Could you check a few things on this model? Use its own coordinates, in mm. Face numbers are marked on the shaded views. A direction names the side the tool comes from. Coordinates: 2 decimals unless noted, no trailing zeros. Write each loop counter-clockwise with the first axis right and the second up, starting at its lowest first coordinate (ties: lowest second). Pieces come first, ordered by that corner, then holes.
Item 1: I want a section at C-C on x = -18.5. Please give me the cut outline in (y, z).
Item 2: Which directions (+Z, -Z, +X, -X, +Y, -Y) give clear straight access to the entire face, cutting with the end or side of a thin tool? Please do the marked faces 4 and 5.
Item 3: If I drill on probe 1 along X at (y, z) = (-8, -2.25); probe 2 along X at (y, z) = (17, -2.5); probe 3 along Y at (x, z) = (-27.5, -4), over which ranges is the centre line in solid material (lowest first)?
Item 4: I want a section at D-D on y = -13. Please give me the cut outline in (x, z), then the cut area to 3 significant figures.
Item 5: Thinking about a two-plate mould opening in Y: for the marked faces 1, 2 and 3, which applies, +Y half, -Y half, draft (parallel to the pull), parting line (faces both ways), or undercut?
Item 6: For P1, Ø1.6, axis at y = 20, z = -4.5, coming from the +X side; P2, Ø10, axis at x = 45, y = -15.5, coming from the -Z side; P3, Ø1, axis at x = 29, y = 20, coming from the -Z side; P4, Ø1.5, axis at x = 4, z = -1, coming from the +Y side, each with a flat end and sliding along its axis, tell me the tip position at first contact or that it passes through.
Item 7: I want a section at B-B on y = -6. Please give me the cut outline in (x, z).
Item 8: I want a section at A-A on x = 8. Please give me the cut outline in (y, z).
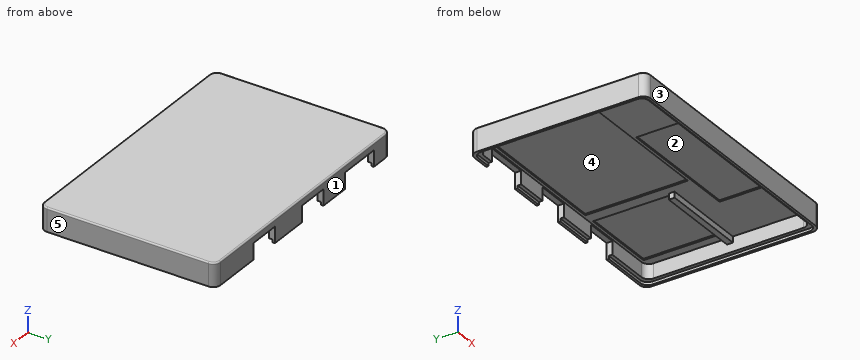
from build123d import *

# Parameters (mm, degrees)
SKETCH_1_W          = 90
SKETCH_1_H          = 60
EXTRUDE_1_DEPTH     = 2
SKETCH_2_W          = 50
SKETCH_2_H          = 35
EXTRUDE_2_DEPTH     = 1
SKETCH_3_W          = 14
SKETCH_3_H          = 13
EXTRUDE_3_DEPTH     = 10
SKETCH_4_W          = 10
SKETCH_4_H          = 12
EXTRUDE_4_DEPTH     = 5
SKETCH_5_W          = 26
SKETCH_5_H          = 26
EXTRUDE_5_DEPTH     = 1
SKETCH_6_W          = 10
SKETCH_6_H          = 10
EXTRUDE_6_DEPTH     = 7
SKETCH_7_W          = 43
SKETCH_7_H          = 18
EXTRUDE_7_DEPTH     = 1
SKETCH_8_W          = 2
SKETCH_8_H          = 60
EXTRUDE_8_DEPTH     = 5
SKETCH_9_W          = 88
SKETCH_9_H          = 2
EXTRUDE_9_DEPTH     = 5
SKETCH_10_W         = 2
SKETCH_10_H         = 58
EXTRUDE_10_DEPTH    = 5
SKETCH_11_W         = 86
SKETCH_11_H         = 2
EXTRUDE_11_DEPTH    = 5
SKETCH_12_W         = 0.8
SKETCH_12_H         = 60
EXTRUDE_12_DEPTH    = 1
SKETCH_13_W         = 89.2
SKETCH_13_H         = 0.8
EXTRUDE_13_DEPTH    = 1
SKETCH_14_W         = 0.8
SKETCH_14_H         = 59.2
EXTRUDE_14_DEPTH    = 1
SKETCH_15_W         = 88.4
SKETCH_15_H         = 0.8
EXTRUDE_15_DEPTH    = 1
SKETCH_16_W         = 11
SKETCH_16_H         = 8
CUT_EXTRUDE_2_DEPTH = 34
SKETCH_17_W         = 11
SKETCH_17_H         = 6
CUT_EXTRUDE_3_DEPTH = 34
SKETCH_18_W         = 15
SKETCH_18_H         = 11
CUT_EXTRUDE_4_DEPTH = 34
SKETCH_19_W         = 30
SKETCH_19_H         = 2
EXTRUDE_16_DEPTH    = 2
SKETCH_20_W         = 43
SKETCH_20_H         = 18
CUT_EXTRUDE_5_DEPTH = 1.5
SKETCH_21_W         = 26
SKETCH_21_H         = 26
CUT_EXTRUDE_6_DEPTH = 1.5
SKETCH_22_W         = 50
SKETCH_22_H         = 35
CUT_EXTRUDE_7_DEPTH = 1.5
FILLET_1_R          = 2.5
FILLET_2_R          = 2.5
FILLET_3_R          = 0.5


with BuildPart() as part:
    # Эскиз1 → Бобышка-Вытянуть1 (new body)
    with BuildSketch(Plane.XY):
        with Locations((11.347826087, -8.739130435)):
            Rectangle(SKETCH_1_W, SKETCH_1_H)
    extrude(amount=EXTRUDE_1_DEPTH)

    # Эскиз2 → Бобышка-Вытянуть2 (add)
    with BuildSketch(Plane(origin=(0, 0, 0), x_dir=(-1, 0, 0), z_dir=(0, 0, -1))):
        with Locations((3.652173913, 0.760869565)):
            Rectangle(SKETCH_2_W, SKETCH_2_H)
    extrude(amount=EXTRUDE_2_DEPTH)

    # Эскиз3 → Бобышка-Вытянуть3 (add)
    with BuildSketch(Plane(origin=(0, 0, -1), x_dir=(-1, 0, 0), z_dir=(0, 0, -1))):
        with Locations((17.652173913, 5.760869565)):
            Rectangle(SKETCH_3_W, SKETCH_3_H)
    extrude(amount=EXTRUDE_3_DEPTH)

    # Эскиз4 → Бобышка-Вытянуть4 (add)
    with BuildSketch(Plane(origin=(0, 0, -1), x_dir=(-1, 0, 0), z_dir=(0, 0, -1))):
        with Locations((-6.347826087, 15.260869565)):
            Rectangle(SKETCH_4_W, SKETCH_4_H)
    extrude(amount=EXTRUDE_4_DEPTH)

    # Эскиз5 → Бобышка-Вытянуть5 (add)
    with BuildSketch(Plane(origin=(0, 0, 0), x_dir=(-1, 0, 0), z_dir=(0, 0, -1))):
        with Locations((-38.347826087, 5.260869565)):
            Rectangle(SKETCH_5_W, SKETCH_5_H)
    extrude(amount=EXTRUDE_5_DEPTH)

    # Эскиз6 → Бобышка-Вытянуть6 (add)
    with BuildSketch(Plane(origin=(0, 0, -1), x_dir=(-1, 0, 0), z_dir=(0, 0, -1))):
        with Locations((-31.347826087, 14.260869565)):
            Rectangle(SKETCH_6_W, SKETCH_6_H)
    extrude(amount=EXTRUDE_6_DEPTH)

    # Эскиз7 → Бобышка-Вытянуть7 (add)
    with BuildSketch(Plane(origin=(0, 0, 0), x_dir=(-1, 0, 0), z_dir=(0, 0, -1))):
        with Locations((-14.606181905, -26.739130435)):
            Rectangle(SKETCH_7_W, SKETCH_7_H)
    extrude(amount=EXTRUDE_7_DEPTH)

    # Эскиз8 → Бобышка-Вытянуть8 (add)
    with BuildSketch(Plane(origin=(0, 0, 0), x_dir=(-1, 0, 0), z_dir=(0, 0, -1))):
        with Locations((-55.347826087, -8.739130435)):
            Rectangle(SKETCH_8_W, SKETCH_8_H)
    extrude(amount=EXTRUDE_8_DEPTH)

    # Эскиз9 → Бобышка-Вытянуть9 (add)
    with BuildSketch(Plane(origin=(0, 0, 0), x_dir=(-1, 0, 0), z_dir=(0, 0, -1))):
        with Locations((-10.347826087, -37.739130435)):
            Rectangle(SKETCH_9_W, SKETCH_9_H)
    extrude(amount=EXTRUDE_9_DEPTH)

    # Эскиз10 → Бобышка-Вытянуть10 (add)
    with BuildSketch(Plane(origin=(0, 0, 0), x_dir=(-1, 0, 0), z_dir=(0, 0, -1))):
        with Locations((32.652173913, -7.739130435)):
            Rectangle(SKETCH_10_W, SKETCH_10_H)
    extrude(amount=EXTRUDE_10_DEPTH)

    # Эскиз11 → Бобышка-Вытянуть11 (add)
    with BuildSketch(Plane(origin=(0, 0, 0), x_dir=(-1, 0, 0), z_dir=(0, 0, -1))):
        with Locations((-11.347826087, 20.260869565)):
            Rectangle(SKETCH_11_W, SKETCH_11_H)
    extrude(amount=EXTRUDE_11_DEPTH)

    # Эскиз12 → Бобышка-Вытянуть12 (add)
    with BuildSketch(Plane(origin=(0, 0, -5), x_dir=(-1, 0, 0), z_dir=(0, 0, -1))):
        with Locations((-55.947826087, -8.739130435)):
            Rectangle(SKETCH_12_W, SKETCH_12_H)
    extrude(amount=EXTRUDE_12_DEPTH)

    # Эскиз13 → Бобышка-Вытянуть13 (add)
    with BuildSketch(Plane(origin=(0, 0, -5), x_dir=(-1, 0, 0), z_dir=(0, 0, -1))):
        with Locations((-10.947826087, -38.339130435)):
            Rectangle(SKETCH_13_W, SKETCH_13_H)
    extrude(amount=EXTRUDE_13_DEPTH)

    # Эскиз14 → Бобышка-Вытянуть14 (add)
    with BuildSketch(Plane(origin=(0, 0, -5), x_dir=(-1, 0, 0), z_dir=(0, 0, -1))):
        with Locations((33.252173913, -8.339130435)):
            Rectangle(SKETCH_14_W, SKETCH_14_H)
    extrude(amount=EXTRUDE_14_DEPTH)

    # Эскиз15 → Бобышка-Вытянуть15 (add)
    with BuildSketch(Plane(origin=(0, 0, -5), x_dir=(-1, 0, 0), z_dir=(0, 0, -1))):
        with Locations((-11.347826087, 20.860869565)):
            Rectangle(SKETCH_15_W, SKETCH_15_H)
    extrude(amount=EXTRUDE_15_DEPTH)

    # Эскиз16 → Вырез-Вытянуть2 (cut)
    with BuildSketch(Plane.XZ.offset(-9.260869565)):
        with Locations((31.347826087, -4.5)):
            Rectangle(SKETCH_16_W, SKETCH_16_H)
    extrude(amount=-CUT_EXTRUDE_2_DEPTH, mode=Mode.SUBTRACT)

    # Эскиз17 → Вырез-Вытянуть3 (cut)
    with BuildSketch(Plane.XZ.offset(-9.260869565)):
        with Locations((6.347826087, -3.5)):
            Rectangle(SKETCH_17_W, SKETCH_17_H)
    extrude(amount=-CUT_EXTRUDE_3_DEPTH, mode=Mode.SUBTRACT)

    # Эскиз18 → Вырез-Вытянуть4 (cut)
    with BuildSketch(Plane.XZ.offset(0.739130435)):
        with Locations((-17.652173913, -6)):
            Rectangle(SKETCH_18_W, SKETCH_18_H)
    extrude(amount=-CUT_EXTRUDE_4_DEPTH, mode=Mode.SUBTRACT)

    # Эскиз19 → Бобышка-Вытянуть16 (add)
    with BuildSketch(Plane(origin=(0, 0, 0), x_dir=(-1, 0, 0), z_dir=(0, 0, -1))):
        with Locations((-39.347826087, -9.239130435)):
            Rectangle(SKETCH_19_W, SKETCH_19_H)
    extrude(amount=EXTRUDE_16_DEPTH)

    # Эскиз20 → Вырез-Вытянуть5 (cut)
    with BuildSketch(Plane(origin=(0, 0, -1), x_dir=(-1, 0, 0), z_dir=(0, 0, -1))):
        with Locations((-14.606181905, -26.739130435)):
            Rectangle(SKETCH_20_W, SKETCH_20_H)
    extrude(amount=-CUT_EXTRUDE_5_DEPTH, mode=Mode.SUBTRACT)

    # Эскиз21 → Вырез-Вытянуть6 (cut)
    with BuildSketch(Plane(origin=(0, 0, -1), x_dir=(-1, 0, 0), z_dir=(0, 0, -1))):
        with Locations((-38.347826087, 5.260869565)):
            Rectangle(SKETCH_21_W, SKETCH_21_H)
    extrude(amount=-CUT_EXTRUDE_6_DEPTH, mode=Mode.SUBTRACT)

    # Эскиз22 → Вырез-Вытянуть7 (cut)
    with BuildSketch(Plane(origin=(0, 0, -1), x_dir=(-1, 0, 0), z_dir=(0, 0, -1))):
        with Locations((3.652173913, 0.760869565)):
            Rectangle(SKETCH_22_W, SKETCH_22_H)
    extrude(amount=-CUT_EXTRUDE_7_DEPTH, mode=Mode.SUBTRACT)

    # Скругление1
    fillet_1_edges = [part.edges().sort_by_distance(p)[0] for p in [
        (54.347826087, -36.739130435, -2.5),
        (-31.652173913, -36.739130435, -2.5),
        (54.347826087, 19.260869565, -2.5),
        (-31.652173913, 19.260869565, -2.5),
        (-33.652173913, 21.260869565, -2),
        (56.347826087, 21.260869565, -2),
        (56.347826087, -38.739130435, -2),
        (-33.652173913, -38.739130435, -2),
    ]]
    fillet(fillet_1_edges, radius=FILLET_1_R)

    # Скругление2
    fillet_2_edges = [part.edges().sort_by_distance(p)[0] for p in [
        (55.547826087, -37.939130435, -5.5),
        (-32.852173913, -37.939130435, -5.5),
        (55.547826087, 20.460869565, -5.5),
        (-32.852173913, 20.460869565, -5.5),
    ]]
    fillet(fillet_2_edges, radius=FILLET_2_R)

    # Скругление3
    fillet_3_edges = [part.edges().sort_by_distance(p)[0] for p in [
        (11.347826087, 21.260869565, 2),
        (56.347826087, -8.739130435, 2),
        (-33.652173913, -8.739130435, 2),
        (11.347826087, -38.739130435, 2),
        (-32.919940866, 20.528636518, 2),
        (-32.919940866, -38.006897388, 2),
        (55.61559304, -38.006897388, 2),
        (55.61559304, 20.528636518, 2),
    ]]
    fillet(fillet_3_edges, radius=FILLET_3_R)


solid = part.part
Response values:
1. outline: (-38.74, -6) - (-37.94, -6) - (-37.94, -5) - (-36.74, -5) - (-36.74, 0) - (-16.74, 0) - (-16.74, 0.5) - (18.26, 0.5) - (18.26, 0) - (19.26, 0) - (19.26, -0.5) - (21.26, -0.5) - (21.26, 1.5) arc R0.5 ccw to (20.76, 2) - (-38.24, 2) arc R0.5 ccw to (-38.74, 1.5) - close
2. face 4: -Z
2. face 5: +Z, -Z, +X, +Y, -Y
3. probe 1: x = -33.65 to -31.65, 54.35 to 56.35
3. probe 2: x = -33.65 to -31.64, 54.34 to 56.35
3. probe 3: y = -38.74 to -36.74, 19.26 to 21.26
4. outline: (-33.65, -6) - (-32.85, -6) - (-32.85, -5) - (-31.65, -5) - (-31.65, 0) - (-28.65, 0) - (-28.65, 0.5) - (21.35, 0.5) - (21.35, 0) - (54.35, 0) - (54.35, -5) - (55.55, -5) - (55.55, -6) - (56.35, -6) - (56.35, 1.5) arc R0.5 ccw to (55.85, 2) - (-33.15, 2) arc R0.5 ccw to (-33.65, 1.5) - close
4. area: 176 mm2
5. face 1: +Y half
5. face 2: undercut
5. face 3: -Y half
6. P1: stops at x = 56.31
6. P2: stops at z = 0
6. P3: stops at z = -0.5
6. P4: stops at y = 21.26
7. outline: (-33.65, -6) - (-32.85, -6) - (-32.85, -5) - (-31.65, -5) - (-31.65, 0) - (-28.65, 0) - (-28.65, 0.5) - (21.35, 0.5) - (21.35, 0) - (25.35, 0) - (25.35, 0.5) - (51.35, 0.5) - (51.35, 0) - (54.35, 0) - (54.35, -5) - (55.55, -5) - (55.55, -6) - (56.35, -6) - (56.35, 1.5) arc R0.5 ccw to (55.85, 2) - (-33.15, 2) arc R0.5 ccw to (-33.65, 1.5) - close
8. outline: (-38.74, -6) - (-37.94, -6) - (-37.94, -5) - (-36.74, -5) - (-36.74, 0) - (-35.74, 0) - (-35.74, 0.5) - (-17.74, 0.5) - (-17.74, 0) - (-16.74, 0) - (-16.74, 0.5) - (18.26, 0.5) - (18.26, 0) - (19.26, 0) - (19.26, -0.5) - (21.26, -0.5) - (21.26, 1.5) arc R0.5 ccw to (20.76, 2) - (-38.24, 2) arc R0.5 ccw to (-38.74, 1.5) - close
